Input: part model. Units: mm. Frame: model coordinates. Give positions to 0.01 mm unless a question says otherwise; leave off trailing zeros. Order: outer loops, then holes, each group sorted by start corner. A loop starts at its lowest first (then second) coordinate and runs counter-clockwise, first axis right, second up. Notation, with made-up numbers: M -12.5,82 L 21.5,82 A25 ccw 21.5,94 Z; hole C 73,-21 d7. An arc over 180 degrees is marked long. Use a Markdown table: item, result.
from build123d import *

# Parameters (mm, degrees)
SKETCH_1_R      = 27.5
SKETCH_1_R_2    = 10
EXTRUDE_1_DEPTH = 10


with BuildPart() as part:
    # Sketch 1 → Extrude 1 (new body)
    with BuildSketch(Plane(origin=(0, 0, 0), x_dir=(1, 0, 0), z_dir=(0, 1, 0))):
        with BuildLine():
            ThreePointArc((36.626693786, -26.14355183), (45, 0), (36.626693786, 26.14355183))
            ThreePointArc((36.626693786, 26.14355183), (35.489388485, 31.722157226), (38.87340923, 36.300661906))
            ThreePointArc((38.87340923, 36.300661906), (42.889809267, 64.52547333), (14.571428571, 61.232941793))
            ThreePointArc((14.571428571, 61.232941793), (0, 52.989280604), (-14.571428571, 61.232941793))
            ThreePointArc((-14.571428571, 61.232941793), (-42.889809267, 64.52547333), (-38.87340923, 36.300661906))
            ThreePointArc((-38.87340923, 36.300661906), (-35.489388485, 31.722157226), (-36.626693786, 26.14355183))
            ThreePointArc((-36.626693786, 26.14355183), (-45, 0), (-36.626693786, -26.14355183))
            ThreePointArc((-36.626693786, -26.14355183), (-35.489388485, -31.722157226), (-38.87340923, -36.300661906))
            ThreePointArc((-38.87340923, -36.300661906), (-42.889809267, -64.52547333), (-14.571428571, -61.232941793))
            ThreePointArc((-14.571428571, -61.232941793), (0, -52.989280604), (14.571428571, -61.232941793))
            ThreePointArc((14.571428571, -61.232941793), (42.889809267, -64.52547333), (38.87340923, -36.300661906))
            ThreePointArc((38.87340923, -36.300661906), (35.489388485, -31.722157226), (36.626693786, -26.14355183))
        make_face()
        with Locations(Location((0, 0, 0), (0, 0, 270))):
            Circle(SKETCH_1_R, mode=Mode.SUBTRACT)
        with Locations(Location((30, -51.961524227, 0), (0, 0, 270))):
            Circle(SKETCH_1_R_2, mode=Mode.SUBTRACT)
        with Locations(Location((-30, -51.961524227, 0), (0, 0, 90))):
            Circle(SKETCH_1_R_2, mode=Mode.SUBTRACT)
        with Locations(Location((-30, 51.961524227, 0), (0, 0, 270))):
            Circle(SKETCH_1_R_2, mode=Mode.SUBTRACT)
        with Locations(Location((30, 51.961524227, 0), (0, 0, 90))):
            Circle(SKETCH_1_R_2, mode=Mode.SUBTRACT)
    extrude(amount=EXTRUDE_1_DEPTH)


solid = part.part
1) Cut plane B-B on z = 0. Return loops of the section in (x, y), and give its area (3 significant figures).
Response values:
| item | result |
|---|---|
| outline | M -45,0 L -27.5,0 L -27.5,10 L -45,10 Z; M 27.5,0 L 45,0 L 45,10 L 27.5,10 Z |
| area | 350 mm² |
2) Material intervals for line 1 (X direction, y = 6, z = -51.5); line 2 (Z direction, x = 41, y = 6); line 3 (Z direction, x = 40.5, y = 2), sorted ascending. Write a range as from..to.
Response values:
| item | result |
|---|---|
| line 1 | x = -47.99..-39.99, -20.01..20.01, 39.99..47.99 |
| line 2 | z = -66.21..-37.71, -18.55..18.55, 37.71..66.21 |
| line 3 | z = -66.58..-37.34, -19.62..19.62, 37.34..66.58 |
3) Cut plane C-C on y = 5. Return loops of the section in (x, z).
Response values:
| item | result |
|---|---|
| outline | M -38.87,-36.3 A18 ccw long -14.57,-61.23 A17 cw 14.57,-61.23 A18 ccw long 38.87,-36.3 A7 cw 36.63,-26.14 A45 ccw 36.63,26.14 A7 cw 38.87,36.3 A18 ccw long 14.57,61.23 A17 cw -14.57,61.23 A18 ccw long -38.87,36.3 A7 cw -36.63,26.14 A45 ccw -36.63,-26.14 A7 cw Z; hole C -30,-51.96 d20; hole C -30,51.96 d20; hole C 0,0 d55; hole C 30,-51.96 d20; hole C 30,51.96 d20 |
4) First-contact query: pin 1 Ø4 at (x, y) = (-33.5, 1) entering from -Z; pin 2 Ø2 at (x, y) = (8.5, 3) entering from -Z; pin 3 Ø6 at (y, z) = (2, -28.5) entering from +X; pin 4 Ø12 at (x, z) = (-30, -51.96) entering from -Y. Flat tips, straight axial feed; report the tip coordinate or a pass-through.
Response values:
| item | result |
|---|---|
| pin 1 | stops at z = -69.9 |
| pin 2 | stops at z = -55.89 |
| pin 3 | stops at x = 37.08 |
| pin 4 | passes through |
5) Mould query, pull axis X, two halves, no side actions, for faces 1 (the face through (-0.25, 4.93, 52.99)), 2 (the face through (-38.872, 4.93, -47.347)), 3 (the face through (-22, 10, -17)), 4 (the face through (35.47, 4.93, -31.64)). Classes: released by +X, released by -X, zero draft, split by the parting line, or undercut.
Response values:
| item | result |
|---|---|
| face 1 | undercut |
| face 2 | undercut |
| face 3 | zero draft |
| face 4 | released by +X |
6) Cut plane D-D on x = 0. Return loops of the section in (y, z), and give its area (3 significant figures).
Response values:
| item | result |
|---|---|
| outline | M 0,-52.99 L 10,-52.99 L 10,-27.5 L 0,-27.5 Z; M 0,27.5 L 10,27.5 L 10,52.99 L 0,52.99 Z |
| area | 510 mm² |
7) Cut plane A-A on x = -30. Return loops of the section in (y, z), and give its area (3 significant figures).
Response values:
| item | result |
|---|---|
| outline | M 0,-69.96 L 10,-69.96 L 10,-61.96 L 0,-61.96 Z; M 0,-41.96 L 10,-41.96 L 10,41.96 L 0,41.96 Z; M 0,61.96 L 10,61.96 L 10,69.96 L 0,69.96 Z |
| area | 999 mm² |
